```python
from build123d import *

# Parameters (mm, degrees)
F1_DEPTH = 15.875


with BuildPart() as f1:
    # F0 (on Front) → F1 (new body)
    with BuildSketch(Plane.XZ):
        with BuildLine():
            Line((1059.485458, 522.484738), (-70.814542, 522.484738))
            Line((-70.814542, 522.484738), (-70.814542, -214.115262))
            Line((-70.814542, -214.115262), (233.985458, -214.115262))
            ThreePointArc((233.985458, -214.115262), (269.906482, -199.236287), (284.785458, -163.315262))
            Line((284.785458, -163.315262), (284.785458, -42.665262))
            ThreePointArc((284.785458, -42.665262), (494.335458, 166.884738), (703.885458, -42.665262))
            Line((703.885458, -42.665262), (703.885458, -163.315262))
            ThreePointArc((703.885458, -163.315262), (718.764433, -199.236287), (754.685458, -214.115262))
            Line((754.685458, -214.115262), (1059.485458, -214.115262))
            Line((1059.485458, -214.115262), (1059.485458, 522.484738))
        make_face()
    extrude(amount=F1_DEPTH)


solid = f1.part
```
Design review of the part built by this model. Coordinates are the model's own, in mm. A direction names the side the tool comes from. Give positions to 0.01 mm unless a question says otherwise; leave off trailing zeros. Order: outer loops, then holes, each group sorted by start corner. A loop starts at its lowest first (then second) coordinate and runs counter-clockwise, first axis right, second up. Notation, with made-up numbers: M 86.25,74 L 114.25,74 A34 cw 114.25,108 Z; hole C 74.5,81.5 d3. An arc over 180 degrees is marked long. One line per question, with ' | ' between items. Start each with the question number.
Q1. We need section B-B (z = -70.5). Write out the cut boundary in (x, y) (3 decimals).
Q2. We need section C-C (z = 19.5). Write out the cut boundary in (x, y) (3 decimals).
Q3. We need section D-D (x = 685.5). Write out the cut boundary in (y, z) (3 decimals), plus the area to 3 significant figures.
Q4. For L1, parallel to X at y = -8.25, z = -141; L2, parallel to Z at x = 498, y = -7.25; L3, parallel to X at y = -11.25, z = 59.5, list the stretches that pass through material, from the lowest coordinate up. Write a range as [from, to].
Q5. Machinability: for faces 3 (the face through (486, 0, 241)), 4 (the face through (718.37, -7.83, -198.84)), which of the approach directions +Z, -Z, +X, -X, +Y, -Y give a long, thin tool a straight path to every point of the face, cutting with its end or side? Answer none if there is none.
Q6. We need section A-A (y = -11.5). Write out the cut boundary in (x, z).
Q7. For pin 1 Ø2 at (x, z) = (217.5, -129) entering from +Y, flat-tipped, find the tip position at first contact; note if it passes through.
Q8. The part is to be moulded in two halves that separate along X. For faces 1 (the face through (486, -15.875, 241)), 2 (the face through (269.51, -7.83, -199.63)), say which applies: +X half, -X half, draft (parallel to the pull), parting line (faces both ways), or undercut.
Returned:
1) outline: M -70.815,-15.875 L 284.785,-15.875 L 284.785,0 L -70.815,0 Z; M 703.885,-15.875 L 1059.485,-15.875 L 1059.485,0 L 703.885,0 Z
2) outline: M -70.815,-15.875 L 294.219,-15.875 L 294.219,0 L -70.815,0 Z; M 694.452,-15.875 L 1059.485,-15.875 L 1059.485,0 L 694.452,0 Z
3) outline: M -15.875,43.168 L 0,43.168 L 0,522.485 L -15.875,522.485 Z | area: 7,610 mm2
4) L1: [-70.81, 284.79], [703.89, 1059.49] | L2: [166.85, 522.48] | L3: [-70.81, 311.38], [677.29, 1059.49]
5) face 3: +Z, -Z, +X, -X, +Y | face 4: -Z, +Y, -Y
6) outline: M -70.81,-214.12 L 233.99,-214.12 A50.8 ccw 284.79,-163.32 L 284.79,-42.67 A209.55 cw 703.89,-42.67 L 703.89,-163.32 A50.8 ccw 754.69,-214.12 L 1059.49,-214.12 L 1059.49,522.48 L -70.81,522.48 Z
7) pin 1: y = 0
8) face 1: draft | face 2: undercut
